from build123d import *

# Parameters (mm, degrees)
F1_DEPTH = 5


with BuildPart() as f1:
    # F0 (on Top) → F1 (new body)
    with BuildSketch(Plane.XY):
        with BuildLine():
            Line((1.7, 3.895189), (3, 6.873864))
            ThreePointArc((3, 6.873864), (0, 7.5), (-3, 6.873864))
            Line((-3, 6.873864), (-1.7, 3.895189))
            ThreePointArc((-1.7, 3.895189), (0, 4.25), (1.7, 3.895189))
        make_face()
        with BuildLine():
            ThreePointArc((6.873864, -3), (7.341797, -1.532322), (7.5, 0))
            ThreePointArc((7.5, 0), (7.341797, 1.532322), (6.873864, 3))
            Line((6.873864, 3), (3.895189, 1.7))
            ThreePointArc((3.895189, 1.7), (4.160352, 0.868316), (4.25, 0))
            ThreePointArc((4.25, 0), (4.160352, -0.868316), (3.895189, -1.7))
            Line((3.895189, -1.7), (6.873864, -3))
        make_face()
        with BuildLine():
            ThreePointArc((-3, -6.873864), (0, -7.5), (3, -6.873864))
            Line((3, -6.873864), (1.7, -3.895189))
            ThreePointArc((1.7, -3.895189), (0, -4.25), (-1.7, -3.895189))
            Line((-1.7, -3.895189), (-3, -6.873864))
        make_face()
        with BuildLine():
            Line((-3.895189, 1.7), (-6.873864, 3))
            ThreePointArc((-6.873864, 3), (-7.5, 0), (-6.873864, -3))
            Line((-6.873864, -3), (-3.895189, -1.7))
            ThreePointArc((-3.895189, -1.7), (-4.25, 0), (-3.895189, 1.7))
        make_face()
        with BuildLine():
            ThreePointArc((4.25, 0), (4.160352, 0.868316), (3.895189, 1.7))
            ThreePointArc((3.895189, 1.7), (3.005204, 3.005204), (1.7, 3.895189))
            ThreePointArc((1.7, 3.895189), (0, 4.25), (-1.7, 3.895189))
            ThreePointArc((-1.7, 3.895189), (-3.005204, 3.005204), (-3.895189, 1.7))
            ThreePointArc((-3.895189, 1.7), (-4.25, 0), (-3.895189, -1.7))
            ThreePointArc((-3.895189, -1.7), (-3.005204, -3.005204), (-1.7, -3.895189))
            ThreePointArc((-1.7, -3.895189), (0, -4.25), (1.7, -3.895189))
            ThreePointArc((1.7, -3.895189), (3.005204, -3.005204), (3.895189, -1.7))
            ThreePointArc((3.895189, -1.7), (4.160352, -0.868316), (4.25, 0))
        make_face()
    extrude(amount=F1_DEPTH)


solid = f1.part
Geometry check sheet. Reference: the model listing, model coordinates, mm. A direction names the side the tool comes from. Coordinates: 2 decimals unless noted, no trailing zeros. Order: outer loops, then holes, each group sorted by start corner. A loop starts at its lowest first (then second) coordinate and runs counter-clockwise, first axis right, second up. Notation, with made-up numbers: (34.5, 66.25) -> (50.5, 66.25) arc R15 ccw to (50.5, 88.25) -> close; hole circle Ø2 at (86.5, 3). An arc over 180 degrees is marked (long way). Use a Markdown table: item, result. Add a question column.
1. Cross-section at A-A (z = 4.05). Enter the section's corners in (x, y), and give its area (3 significant figures).
2. Cross-section at D-D (y = 5.5). Enter the section's corners in (x, z).
3. Cross-section at B-B (x = -2.25). Enter the section's corners in (y, z).
4. Go/stop test with flat-tipped pins: pin 1 Ø1 at (x, z) = (-1.5, 2.5) entering from +Y; pin 2 Ø1.5 at (x, z) = (5.5, 3) entering from +Y. Record where each tip stops, or that it passes through.
5. Material ranges on L1, parallel to Y at x = 2.5, z = 0.85; L2, parallel to Y at x = -2.75, z = 1.6; L3, parallel to Y at x = -0.25, z = 0.5, recorded low to high.
6. Cross-section at C-C (y = -2.5). Enter the section's corners in (x, z).
7. Mould release check, pull along X, two halves, no side actions. Record for faces 1 (the face through (0, 0, 5)), 2 (the face through (-5.36, 2.34, 2.46)), 3 (the face through (-2.34, -5.36, 2.46)): pulls with the +X half, pulls with the -X half, needs draft (parallel to the pull), parting line crosses it, or undercut.
8. Set-up check for faces 4 (the face through (2.36, -5.41, 2.46)), 5 (the face through (-2.36, 5.41, 2.46)), 6 (the face through (5.41, 2.36, 2.46)), 7 (the face through (-5.41, -2.36, 2.46)), 8 (the face through (2.99, -3.02, 2.46)): record each of +Z, -Z, +X, -X, +Y, -Y from which the full face is reachable in a straight line by a thin tool's end or side.
Filled sheet:
| question | item | result |
|---|---|---|
| 1 | outline | (-6.87, -3) -> (-3.9, -1.7) arc R4.25 ccw to (-1.7, -3.9) -> (-3, -6.87) arc R7.5 ccw to (3, -6.87) -> (1.7, -3.9) arc R4.25 ccw to (3.9, -1.7) -> (6.87, -3) arc R7.5 ccw to (7.5, 0) arc R7.5 ccw to (6.87, 3) -> (3.9, 1.7) arc R4.25 ccw to (1.7, 3.9) -> (3, 6.87) arc R7.5 ccw to (-3, 6.87) -> (-1.7, 3.9) arc R4.25 ccw to (-3.9, 1.7) -> (-6.87, 3) arc R7.5 ccw to start |
| 1 | area | 120 mm2 |
| 2 | outline | (-2.4, 0) -> (2.4, 0) -> (2.4, 5) -> (-2.4, 5) -> close |
| 3 | outline | (-7.15, 0) -> (-5.16, 0) -> (-5.16, 5) -> (-7.15, 5) -> close; (-3.61, 0) -> (3.61, 0) -> (3.61, 5) -> (-3.61, 5) -> close; (5.16, 0) -> (7.15, 0) -> (7.15, 5) -> (5.16, 5) -> close |
| 4 | pin 1 | y = 7.43 |
| 4 | pin 2 | y = 2.73 |
| 5 | L1 | -7.07 to -5.73, -3.44 to 3.44, 5.73 to 7.07 |
| 5 | L2 | -6.98 to -6.3, -3.24 to 3.24, 6.3 to 6.98 |
| 5 | L3 | -7.5 to 7.5 |
| 6 | outline | (-7.07, 0) -> (-5.73, 0) -> (-5.73, 5) -> (-7.07, 5) -> close; (-3.44, 0) -> (3.44, 0) -> (3.44, 5) -> (-3.44, 5) -> close; (5.73, 0) -> (7.07, 0) -> (7.07, 5) -> (5.73, 5) -> close |
| 7 | face 1 | needs draft |
| 7 | face 2 | undercut |
| 7 | face 3 | pulls with the -X half |
| 8 | face 4 | +Z, -Z, +X |
| 8 | face 5 | +Z, -Z, -X |
| 8 | face 6 | +Z, -Z, +Y |
| 8 | face 7 | +Z, -Z, -Y |
| 8 | face 8 | +Z, -Z |
